Check sheet for the modelled part. Datum: model origin and axes. Units: mm. Face numbers are marked on the shaded views. Give positions to 0.01 mm unless a question says otherwise; leave off trailing zeros. Order: outer loops, then holes, each group sorted by start corner. A loop starts at its lowest first (then second) coordinate and runs counter-clockwise, first axis right, second up. Notation, with made-up numbers: M -23.5,63.25 L 10.5,63.25 A14 cw 10.5,74.25 Z; hole C 68,-12.5 d10. An arc over 180 degrees is marked long. One line per question, with ' | ' between items. Start each with the question number.
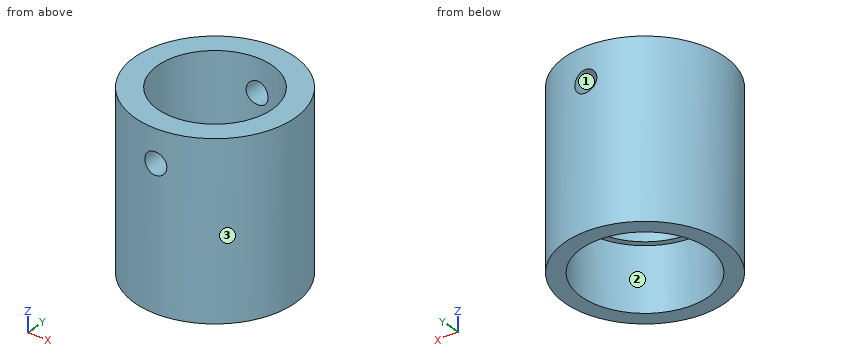
Autodesk Inventor part; units mm, degrees
ref_plane "YZ Plane" through (0, 0, 0) normal (1, 0, 0) x (0, 1, 0)
ref_plane "XZ Plane" through (0, 0, 0) normal (0, 1, 0) x (-1, 0, 0)
ref_plane "XY Plane" through (0, 0, 0) normal (0, 0, 1) x (1, 0, 0)
sketch "草图1" plane through (0, 0, 0) normal (0, 0, 1) x (1, 0, 0)
  circle A0 centre (0, 0) radius 11.5
  circle A1 centre (0, 0) radius 14.5
  dimension "d0" = 23
  dimension "d1" = 3
extrude "拉伸1" add sketch "草图1" along normal blind 11.5
sketch "草图2" plane through (0, 0, 11.5) normal (0, 0, 1) x (1, 0, 0)
  circle A0 centre (0, 0) radius 10.4
  circle A1 centre (0, 0) radius 14.5
  dimension "d4" = 20.8
extrude "拉伸2" add sketch "草图2" along normal blind 20
sketch "草图3" plane through (0, 0, 0) normal (0, 1, 0) x (-1, 0, 0)
  circle A0 centre (0, 25.5367) radius 2
  point P0 (0, 0)
  dimension "d10" = 4
extrude "拉伸3" cut sketch "草图3" along normal mid plane 37.75
properties part number "卡管1_3D 打印"
Item 1: Section check C-C, the plane z = 25. Record the cut outline in (x, y), then the cut area to 3 significant figures.
Item 2: Section check D-D, the plane x = 4.5. Record the cut outline in (y, z).
Item 3: Section check A-A, the plane y = 0. Record the cut outline in (x, z), then the cut area to 3 significant figures.
Item 4: Scan lines: probe 1 along Z at (x, y) = (0, 13.6); probe 2 along Z at (x, y) = (0, -11.2); probe 3 along Z at (x, y) = (10.25, -2). Record each from-to range of solid material in increasing order. Write a range as [from, to].
Item 5: Section check B-B, the plane x = 0. Record the cut outline in (y, z).
Item 6: Go/stop test with flat-tipped pins: P1, Ø5, axis at x = -7.5, z = 21.5, coming from the -Y side; P2, Ø12, axis at x = -10.5, z = 18.5, coming from the -Y side; P3, Ø11.5, axis at x = -1.5, y = -3, coming from the -Z side; P4, Ø4, axis at x = 10, z = 12.5, coming from the -Y side. Record where each tip stops, or that it passes through.
Item 7: Draft check along Y on the marked faces 1, 2 and 3. Enter one of: released by +Y, released by -Y, zero draft, split by the parting line, or undercut.
Reported:
1) outline: M -1.93,-14.37 L -1.93,-10.22 A10.4 cw -1.93,10.22 L -1.93,14.37 A14.5 ccw Z; M 1.93,-14.37 A14.5 ccw 1.93,14.37 L 1.93,10.22 A10.4 cw 1.93,-10.22 Z | area: 289 mm^2
2) outline: M -13.78,0 L -10.58,0 L -10.58,11.5 L -9.38,11.5 L -9.38,31.5 L -13.78,31.5 Z; M 9.38,11.5 L 10.58,11.5 L 10.58,0 L 13.78,0 L 13.78,31.5 L 9.38,31.5 Z
3) outline: M -14.5,0 L -11.5,0 L -11.5,11.5 L -10.4,11.5 L -10.4,31.5 L -14.5,31.5 Z; M 10.4,11.5 L 11.5,11.5 L 11.5,0 L 14.5,0 L 14.5,31.5 L 10.4,31.5 Z | area: 233 mm^2
4) probe 1: z = [0, 23.54], [27.54, 31.5] | probe 2: z = [11.5, 23.54], [27.54, 31.5] | probe 3: z = [11.5, 31.5]
5) outline: M -14.5,0 L -11.5,0 L -11.5,11.5 L -10.4,11.5 L -10.4,23.54 L -14.5,23.54 Z; M -14.5,27.54 L -10.4,27.54 L -10.4,31.5 L -14.5,31.5 Z; M 10.4,11.5 L 11.5,11.5 L 11.5,0 L 14.5,0 L 14.5,23.54 L 10.4,23.54 Z; M 10.4,27.54 L 14.5,27.54 L 14.5,31.5 L 10.4,31.5 Z
6) P1: stops at y = -13.61 | P2: stops at y = -13.78 | P3: passes through | P4: stops at y = -12.09
7) face 1: zero draft | face 2: undercut | face 3: split by the parting line
